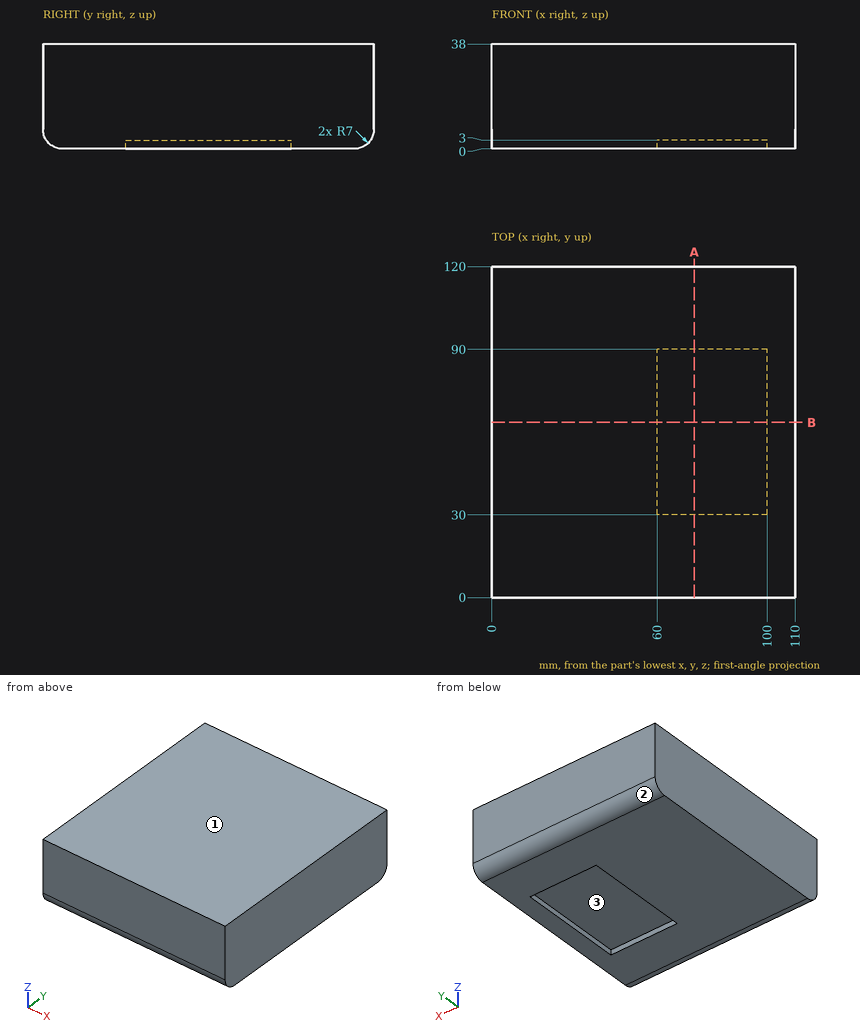
Study the drawing (mm; zero at the part's minimum x, y, z) and answer. Coordinates: 2 decimals unless noted, no trailing zeros. Order: outer loops, then holes, each group sorted by start corner. A loop starts at its lowest first (then second) coordinate and runs counter-clockwise, first axis right, second up. Notation, with made-up numbers: (-11, 85) -> (18, 85) arc R25 cw to (18, 112) -> close; hole circle Ø1 at (80, 52.5). An arc over 180 degrees is marked (long way). Answer in a Markdown table with one row per item. Add a question column.
Item 1: Each of these flat-tipped pins is pushed along its axis until it touches: P1, Ø6, axis at y = 104.5, z = 18, coming from the -X side; P2, Ø3.5, axis at x = 80, z = 1.5, coming from the +Y side; P3, Ø3.5, axis at x = 76, z = 1, coming from the -Y side. Where does it stop, or does it pass through?
Item 2: Determine the mould class of the marked faces 1, 2 and 3 for opening direction Y: +Y half, -Y half, draft (parallel to the pull), parting line (faces both ways), or undercut.
Item 3: Find the intervals of material crossed by L1, parallel to Z at x = 90, y = 35, in increasing order. Write a range as from..to.
Item 4: Find section A-A (x = 73.5). Write down the section's boundary in (y, z).
Item 5: Find section B-B (y = 63.5). Write down the section's boundary in (x, z), then the cut area to 3 significant figures.
Result set:
| question | item | result |
|---|---|---|
| 1 | P1 | stops at x = 0 |
| 1 | P2 | stops at y = 118.91 |
| 1 | P3 | stops at y = 1.44 |
| 2 | face 1 | draft |
| 2 | face 2 | +Y half |
| 2 | face 3 | undercut |
| 3 | L1 | z = 3..38 |
| 4 | outline | (0, 7) arc R7 ccw to (7, 0) -> (30, 0) -> (30, 3) -> (90, 3) -> (90, 0) -> (113, 0) arc R7 ccw to (120, 7) -> (120, 38) -> (0, 38) -> close |
| 5 | outline | (0, 0) -> (60, 0) -> (60, 3) -> (100, 3) -> (100, 0) -> (110, 0) -> (110, 38) -> (0, 38) -> close |
| 5 | area | 4,060 mm² |
